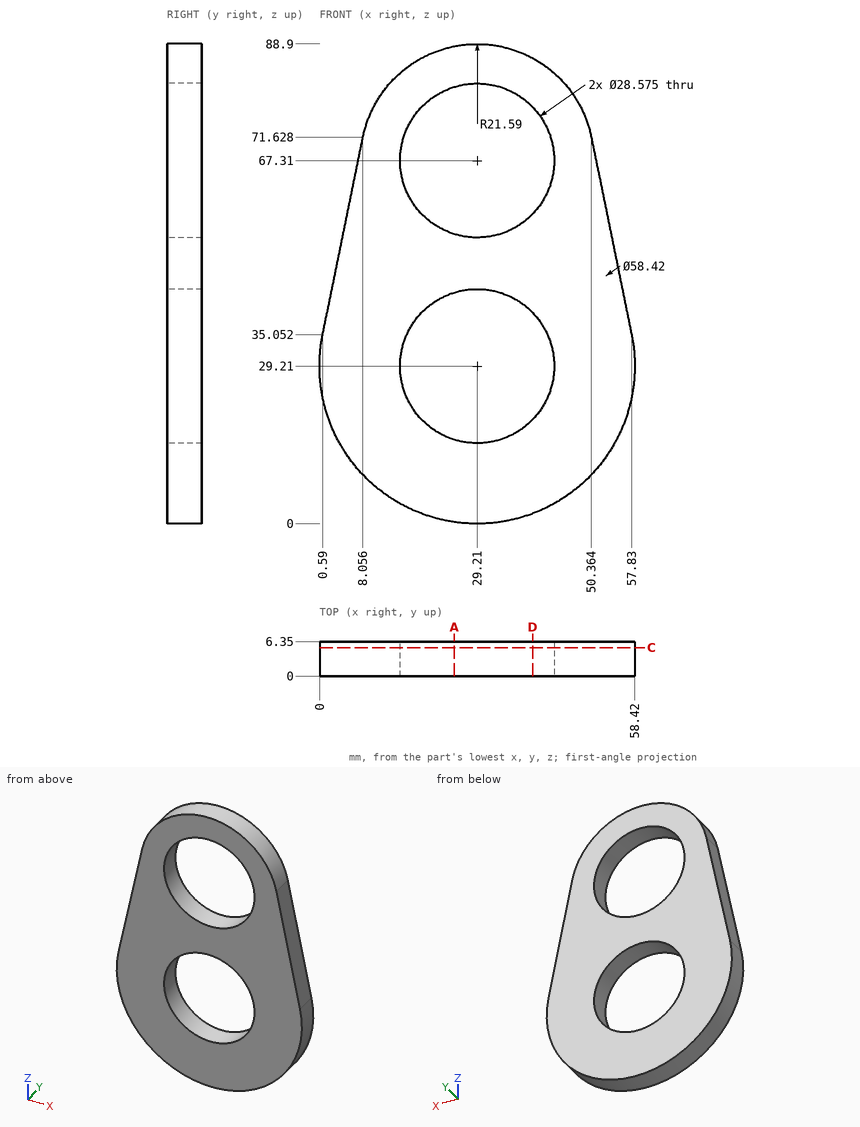
Could you check a few things on this drawing? It's one solid part, dimensions in mm from its lowest x, y, z. Round coordinates to 2 decimals unless told otherwise and drop trailing zeros. Loops run counter-clockwise (first coordinate to the right, second up) from the corner with the lowest first, then second, coordinate; pieces in that order, holes last. Notation, with made-up numbers: (2.25, -9.5) -> (60.25, -9.5) arc R20 ccw to (60.25, 2.5) -> close; hole circle Ø6 at (42.5, -6). An arc over 180 degrees is marked (long way). Answer as CSV lines item,"result".
1. If we section it at A-A on x = 25: Count the separate pieces of the cut face and the enclosed holes in it, plus the area to 3 significant figures.
Final values:
separate pieces,"3"
enclosed holes,"0"
area,"213 mm^2"
2. If we section it at D-D on x = 39.5: Please give me the cut outline in (y, z), plus the area to 3 significant figures.
Final values:
outline,"(0, 1.87) -> (6.35, 1.87) -> (6.35, 19.3) -> (0, 19.3) -> close; (0, 39.12) -> (6.35, 39.12) -> (6.35, 57.4) -> (0, 57.4) -> close; (0, 77.22) -> (6.35, 77.22) -> (6.35, 86.29) -> (0, 86.29) -> close"
area,"284 mm^2"
3. If we section it at C-C on y = 5.25: Please give me the cut outline in (x, z) (1 decimal), plus the area to 3 significant figures.
Final values:
outline,"(0.6, 35.1) arc R29.2 ccw (long way) to (57.8, 35.1) -> (50.4, 71.6) arc R21.6 ccw to (8.1, 71.6) -> close; hole circle Ø28.6 at (29.2, 29.2); hole circle Ø28.6 at (29.2, 67.3)"
area,"2,760 mm^2"
4. If I drill on L1, parallel to Z at x = 23, y = 2; L2, parallel to Z at x = 38, y = 2.5 (1 decimal); L3, parallel to X at y = 2.5, z = 75.5, over which ranges is the centre line in solid material (lowest first)?
Final values:
L1,"z = 0.67 to 16.34, 42.08 to 54.44, 80.18 to 87.99"
L2,"z = 1.4 to 17.9, 40.5 to 56, 78.6 to 87"
L3,"x = 9.23 to 17.5, 40.92 to 49.19"
5. For pin 1 (3 mm diameter, centred on x = 24, y = 4.5, fed in from +Z); pin 2 (1.5 mm diameter, centred on x = 17.5, y = 2, fed in from +Z); pin 3 (2 mm diameter, centred on x = 36, y = 4, fed in from -Z), each with a flat end and sliding along its axis, tell me the tip position at first contact or that it passes through.
Final values:
pin 1,"stops at z = 88.58"
pin 2,"stops at z = 85.91"
pin 3,"stops at z = 0.58"
